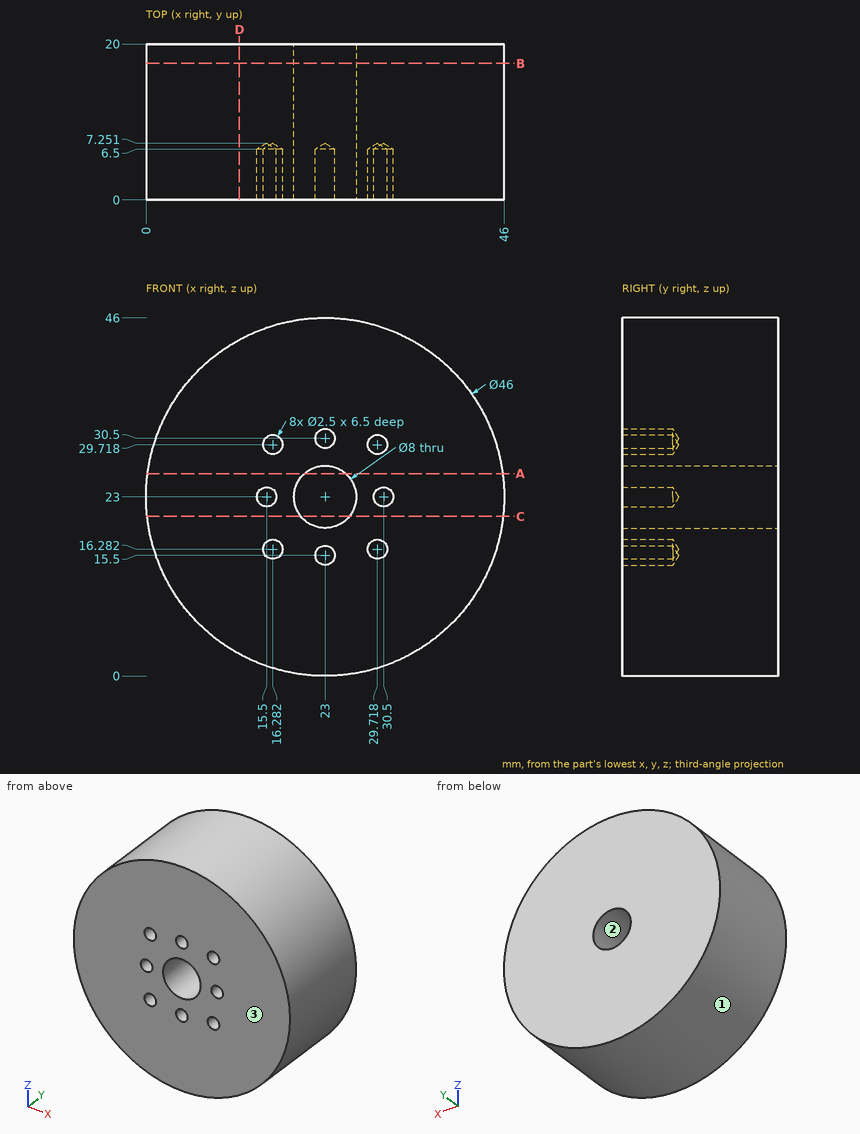
Job drawing, mm, ordinate dimensions from the low corner. One solid piece. Give positions to 0.01 mm unless a question says otherwise; leave off trailing zeros. Loops run counter-clockwise (first coordinate to the right, second up) from the corner with the lowest first, then second, coordinate; pieces in that order, holes last. Notation, with made-up numbers: (21, 77) -> (33, 77) arc R9 cw to (33, 94) -> close; hole circle Ø7 at (-9.75, -7). An arc over 180 degrees is marked (long way). Write each question's results on one line, items separated by ' | '. Start each with the question number.
Q1. Band-saw the part on D-D on x = 12. List the corners of the cut face in (y, z).
Q2. Band-saw the part on A-A on z = 26. List the corners of the cut face in (x, y) (1 decimal).
Q3. Wall check: L1, parallel to X at y = 3, z = 23; L2, parallel to X at y = 3, z = 23.5 (1 decimal). Give the ranges that are in metal, low to high.
Q4. Pin check, flat tips, straight feed: P1, Ø12, axis at y = 18, z = 39.5, coming from the +X side; P2, Ø4, axis at x = 18.5, y = 16, coming from the -Z side; P3, Ø12, axis at x = 36.5, y = 9, coming from the +Z side. Stop position of each tip, or through.
Q5. Band-saw the part on C-C on z = 20.5. List the corners of the cut face in (x, y).
Q6. Band-saw the part on B-B on y = 17.5. List the corners of the cut face in (x, z), plus the area to 3 significant figures.
Q7. Pull direction X, two halves, no side cores. Call the marked faces 1, 2 and 3: +X half, -X half, draft (parallel to the pull), parting line (faces both ways), or undercut.
Results are:
1) outline: (0, 2.8) -> (20, 2.8) -> (20, 43.2) -> (0, 43.2) -> close
2) outline: (0.2, 0) -> (20.4, 0) -> (20.4, 20) -> (0.2, 20) -> close; (25.6, 0) -> (45.8, 0) -> (45.8, 20) -> (25.6, 20) -> close
3) L1: x = 0 to 14.25, 16.75 to 19, 27 to 29.25, 31.75 to 46 | L2: x = 0 to 14.4, 16.6 to 19, 27 to 29.4, 31.6 to 46
4) P1: stops at x = 43.46 | P2: stops at z = 0.14 | P3: stops at z = 44.74
5) outline: (0.14, 0) -> (19.88, 0) -> (19.88, 20) -> (0.14, 20) -> close; (26.12, 0) -> (45.86, 0) -> (45.86, 20) -> (26.12, 20) -> close
6) outline: circle Ø46 at (23, 23); hole circle Ø8 at (23, 23) | area: 1,610 mm²
7) face 1: parting line | face 2: undercut | face 3: draft
